Part model, mm, in its own coordinate system. A direction names the side the tool comes from. Coordinates: 2 decimals unless noted, no trailing zeros. Loops run counter-clockwise (first coordinate to the right, second up) from the corner with the lowest first, then second, coordinate; pieces in that order, holes last. Notation, with made-up numbers: (34.5, -4) - (54.5, -4) arc R6 ccw to (54.5, 6) - close; hole circle Ø8 at (-24, 41.5). An arc over 180 degrees is marked (long way). Use a Markdown table: item, result. Add a question column.
1) Pull direction Y, two halves, no side cores. Call faces 1 (the face through (-1.73, 15.49, -7.81)), 2 (the face through (4, 0, -2)), 3 (the face through (-2, 15, -6)), 4 (the face through (-6, 11, 0)): +Y half, -Y half, draft (parallel to the pull), parting line (faces both ways), or undercut.
2) Band-saw the part on B-B (z = 0). Give the cut face in (x, y), plus the area to 3 significant figures.
3) Band-saw the part on C-C (y = 11.75). Give the cut face in (x, z).
4) Band-saw the part on D-D (x = -6.25). Give the cut face in (y, z).
5) Band-saw the part on A-A (x = 0). Give the cut face in (y, z).
6) Tool access for faces 5 (the face through (-2, 7, -6)), 6 (the face through (-4, 16, 2)): list every direction of +Z, -Z, +X, -X, +Y, -Y with a clear straight run to the whole face (end or side of a thin tool).
7) Drop flat-ended pins along their axis: P1, Ø1.5, axis at y = 12, z = -1, coming from the +X side; P2, Ø1, axis at x = -3.5, y = 5.5, coming from the +Z side; P3, Ø1, axis at x = -1.5, y = 12, coming from the -Z side. Give the stop position or say it passes through.
8) Probe probe 1 along Y at (x, z) = (6.25, -3.5); probe 2 along X at (y, z) = (15.7, 0). List the from-to ranges inside material, lowest first. Write a range as [from, to].
Autodesk Inventor part; units mm, degrees
ref_plane "YZ Plane" through (0, 0, 0) normal (1, 0, 0) x (0, 1, 0)
ref_plane "XZ Plane" through (0, 0, 0) normal (0, 1, 0) x (-1, 0, 0)
ref_plane "XY Plane" through (0, 0, 0) normal (0, 0, 1) x (1, 0, 0)
sketch "Sketch1" plane through (0, 0, 0) normal (0, 1, 0) x (-1, 0, 0)
  circle A0 centre (0, 0) radius 8
  circle A1 centre (0, 0) radius 4
  dimension "d0" = 16
  dimension "d1" = 8
extrude "Extrusion1" add sketch "Sketch1" along normal blind 15
sketch "Sketch2" plane through (0, 15, 0) normal (0, 1, 0) x (1, 0, 0)
  circle A0 centre (0, 0) radius 8
  circle A1 centre (0, 0) radius 6
  dimension "d4" = 12
extrude "Extrusion2" cut sketch "Sketch2" against normal blind 8
sketch "Sketch3" plane through (0, 15, 0) normal (0, 1, 0) x (1, 0, 0)
  circle A0 centre (0, 0) radius 4
  circle A1 centre (0, 0) radius 8
  dimension "d7" = 16
extrude "Extrusion3" add sketch "Sketch3" along normal blind 1
properties part number "Timping Pully" material "Aluminum"
Answer block:
| question | item | result |
|---|---|---|
| 1 | face 1 | draft |
| 1 | face 2 | -Y half |
| 1 | face 3 | undercut |
| 1 | face 4 | undercut |
| 2 | outline | (-8, 0) - (-4, 0) - (-4, 16) - (-8, 16) - (-8, 15) - (-6, 15) - (-6, 7) - (-8, 7) - close; (4, 0) - (8, 0) - (8, 7) - (6, 7) - (6, 15) - (8, 15) - (8, 16) - (4, 16) - close |
| 2 | area | 96.0 mm2 |
| 3 | outline | circle Ø12 at (0, 0); hole circle Ø8 at (0, 0) |
| 4 | outline | (0, -4.99) - (7, -4.99) - (7, 4.99) - (0, 4.99) - close; (15, -4.99) - (16, -4.99) - (16, 4.99) - (15, 4.99) - close |
| 5 | outline | (0, -8) - (7, -8) - (7, -6) - (15, -6) - (15, -8) - (16, -8) - (16, -4) - (0, -4) - close; (0, 4) - (16, 4) - (16, 8) - (15, 8) - (15, 6) - (7, 6) - (7, 8) - (0, 8) - close |
| 6 | face 5 | none |
| 6 | face 6 | +Z, -Z, +X, -X, +Y |
| 7 | P1 | x = 5.99 |
| 7 | P2 | z = 7.42 |
| 7 | P3 | z = -5.92 |
| 8 | probe 1 | [0, 7], [15, 16] |
| 8 | probe 2 | [-8, -4], [4, 8] |
